The listing builds one solid part. Answer for the finished solid, in the listing's coordinates (mm). Face numbers are marked on the shaded views. A direction names the side the tool comes from. Coordinates: 2 decimals unless noted, no trailing zeros. Loops run counter-clockwise (first coordinate to the right, second up) from the corner with the lowest first, then second, coordinate; pieces in that order, holes last. Notation, with made-up numbers: (75.25, -26.5) -> (102.25, -26.5) arc R23 cw to (102.25, 2.5) -> close; hole circle Ø8 at (-4.5, 70.25). An arc over 180 degrees is marked (long way). Answer in a Markdown table with one row per item.
```python
from build123d import *

# Parameters (mm, degrees)
M3_TAPPED_HOLE1_D           = 2.5
M3_TAPPED_HOLE1_DEPTH       = 8.5
M3_TAPPED_HOLE1_CSINK_D     = 3.05
M3_TAPPED_HOLE1_CSINK_ANGLE = 120
M3_TAPPED_HOLE1_TIP         = 0.751075774


with BuildPart() as part:
    # Sketch1 → Revolve3 (revolve)
    with BuildSketch(Plane.XY):
        with BuildLine():
            Line((-35, 5), (-31.2, 5))
            Line((-31.2, 5), (-30.969059892, 4.6))
            ThreePointArc((-30.969059892, 4.6), (-30.822649731, 4.453589838), (-30.622649731, 4.4))
            Line((-30.622649731, 4.4), (-30.4, 4.4))
            ThreePointArc((-30.4, 4.4), (-30.117157288, 4.517157288), (-30, 4.8))
            Line((-30, 4.8), (-30, 4.9))
            Line((-30, 4.9), (-29.9, 5))
            Line((-29.9, 5), (-15, 5))
            Line((-15, 5), (-15, 6.5))
            Line((-15, 6.5), (-2, 6.5))
            Line((-2, 6.5), (-2, 9.4))
            Line((-2, 9.4), (0, 9.4))
            Line((0, 9.4), (0, 7.42))
            Line((0, 7.42), (37, 7.42))
            Line((37, 7.42), (37, 4.5))
            Line((37, 4.5), (44, 4.5))
            Line((44, 4.5), (44, 3))
            Line((44, 3), (57, 3))
            Line((57, 3), (57, 2.85))
            Line((57, 2.85), (57.75, 2.85))
            Line((57.75, 2.85), (57.75, 3))
            Line((57.75, 3), (59, 3))
            Line((59, 3), (59.5, 2.5))
            Line((59.5, 2.5), (59.5, 0))
            Line((59.5, 0), (-49.5, 0))
            Line((-49.5, 0), (-49.5, 2.25))
            Line((-49.5, 2.25), (-49.25, 2.5))
            Line((-49.25, 2.5), (-40, 2.5))
            Line((-40, 2.5), (-40, 3.45))
            Line((-40, 3.45), (-39.75, 3.7))
            Line((-39.75, 3.7), (-35.683012702, 3.7))
            ThreePointArc((-35.683012702, 3.7), (-35.506236007, 3.773223305), (-35.433012702, 3.95))
            Line((-35.433012702, 3.95), (-35.433012702, 4.25))
            Line((-35.433012702, 4.25), (-35, 5))
        make_face()
    revolve(axis=Axis((88.99, 0, 0), (-1, 0, 0)))

    # M3 Tapped Hole1
    with Locations(Plane.ZY.offset(49.5)):
        with Locations((0, 0)):
            CounterSinkHole(M3_TAPPED_HOLE1_D / 2, M3_TAPPED_HOLE1_CSINK_D / 2, depth=M3_TAPPED_HOLE1_DEPTH, counter_sink_angle=M3_TAPPED_HOLE1_CSINK_ANGLE)
            with Locations((0, 0, -(M3_TAPPED_HOLE1_DEPTH + M3_TAPPED_HOLE1_TIP / 2))):  # 118° drill point
                Cone(0, M3_TAPPED_HOLE1_D / 2, M3_TAPPED_HOLE1_TIP, mode=Mode.SUBTRACT)


solid = part.part
```
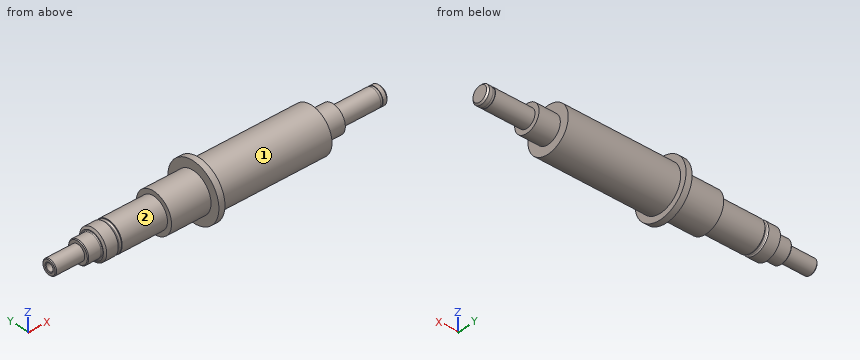
Item 1: A cutting plane is placed at B-B, the plane x = -6. Determine the outline of the cut face in (y, z), plus the area to 3 significant figures.
Findings below:
| item | result |
|---|---|
| outline | circle Ø13 at (0, 0) |
| area | 133 mm2 |
Item 2: A tool of negligible diameter and unlimited length cuts with its end or side. For the marked faces 1 and 2, from which of +Z, -Z, +X, -X, +Y, -Y can it reach the whole face along a straight path? Write none if from no direction.
Findings below:
| item | result |
|---|---|
| face 1 | +X |
| face 2 | -X |
Item 3: A cutting plane is placed at A-A, the plane x = 31. Determine the outline of the cut face in (y, z), plus the area to 3 significant figures.
Findings below:
| item | result |
|---|---|
| outline | circle Ø14.84 at (0, 0) |
| area | 173 mm2 |
Item 4: Flat-ended cylindrical pins translate along their axes: pin 1 Ø3 at (y, z) = (1, -4.5) entering from +X; pin 2 Ø1 at (y, z) = (-2, 7.5) entering from -X; pin 3 Ø6 at (x, z) = (-7.5, 3) entering from -Y. Find the tip coordinate at first contact, or state that the pin passes through.
Findings below:
| item | result |
|---|---|
| pin 1 | stops at x = 44 |
| pin 2 | stops at x = -2 |
| pin 3 | stops at y = -6.5 |
Item 5: Find the intervals of material crossed by probe 1 along Z at (x, y) = (-45.75, 0); probe 2 along X at (y, z) = (2.75, 5), in increasing order.
Findings below:
| item | result |
|---|---|
| probe 1 | z = -2.5 to -1.25, 1.25 to 2.5 |
| probe 2 | x = -15 to 37 |
